```python
from build123d import *

# Parameters (mm, degrees)
F0_R     = 9.4
F1_DEPTH = 3


with BuildPart() as f1:
    # F0 (on Front) → F1 (new body)
    with BuildSketch(Plane.XZ):
        with BuildLine():
            Line((58.8, 11.4), (0, 11.4))
            ThreePointArc((0, 11.4), (-9.870808, 5.703258), (-9.87645, -5.693483))
            Line((-9.87645, -5.693483), (-0.07645, -22.693483))
            Line((-0.07645, -22.693483), (19.523115, -56.692727))
            Line((19.523115, -56.692727), (29.322897, -73.692349))
            ThreePointArc((29.322897, -73.692349), (33.496089, -77.869674), (39.199347, -79.398866))
            Line((39.199347, -79.398866), (156.799347, -79.398866))
            ThreePointArc((156.799347, -79.398866), (166.670155, -73.702124), (166.675796, -62.305384))
            Line((166.675796, -62.305384), (127.47645, 5.693483))
            ThreePointArc((127.47645, 5.693483), (123.303258, 9.870808), (117.6, 11.4))
            Line((117.6, 11.4), (98, 11.4))
            Line((98, 11.4), (58.8, 11.4))
        make_face()
        with Locations((39.199347, -67.998866)):
            Circle(F0_R, mode=Mode.SUBTRACT)
        with Locations((58.799347, -67.998866)):
            Circle(F0_R, mode=Mode.SUBTRACT)
        with Locations((78.399347, -67.998866)):
            Circle(F0_R, mode=Mode.SUBTRACT)
        with Locations((29.399564, -50.999244)):
            Circle(F0_R, mode=Mode.SUBTRACT)
        with Locations((19.599782, -33.999622)):
            Circle(F0_R, mode=Mode.SUBTRACT)
        with Locations((48.999564, -50.999244)):
            Circle(F0_R, mode=Mode.SUBTRACT)
        with Locations((68.599564, -50.999244)):
            Circle(F0_R, mode=Mode.SUBTRACT)
        with Locations((39.199782, -33.999622)):
            Circle(F0_R, mode=Mode.SUBTRACT)
        with Locations((58.799782, -33.999622)):
            Circle(F0_R, mode=Mode.SUBTRACT)
        with Locations((97.999347, -67.998866)):
            Circle(F0_R, mode=Mode.SUBTRACT)
        with Locations((117.599347, -67.998866)):
            Circle(F0_R, mode=Mode.SUBTRACT)
        with Locations((137.199347, -67.998866)):
            Circle(F0_R, mode=Mode.SUBTRACT)
        with Locations((156.799347, -67.998866)):
            Circle(F0_R, mode=Mode.SUBTRACT)
        with Locations((88.199564, -50.999244)):
            Circle(F0_R, mode=Mode.SUBTRACT)
        with Locations((107.799564, -50.999244)):
            Circle(F0_R, mode=Mode.SUBTRACT)
        with Locations((78.399782, -33.999622)):
            Circle(F0_R, mode=Mode.SUBTRACT)
        with Locations((97.999782, -33.999622)):
            Circle(F0_R, mode=Mode.SUBTRACT)
        with Locations((117.599782, -33.999622)):
            Circle(F0_R, mode=Mode.SUBTRACT)
        with Locations((127.399564, -50.999244)):
            Circle(F0_R, mode=Mode.SUBTRACT)
        with Locations((146.999564, -50.999244)):
            Circle(F0_R, mode=Mode.SUBTRACT)
        with Locations((137.199782, -33.999622)):
            Circle(F0_R, mode=Mode.SUBTRACT)
        with BuildLine():
            ThreePointArc((9.8, -26.4), (5.097314, -25.139087), (1.656261, -21.694626))
            ThreePointArc((1.656261, -21.694626), (7.370097, -7.919495), (19.2, -17))
            ThreePointArc((19.2, -17), (16.446804, -23.646804), (9.8, -26.4))
        make_face(mode=Mode.SUBTRACT)
        with Locations((29.4, -17)):
            Circle(F0_R, mode=Mode.SUBTRACT)
        with Locations((49, -17)):
            Circle(F0_R, mode=Mode.SUBTRACT)
        with BuildLine():
            ThreePointArc((76.743739, -12.305374), (77.680505, -14.570097), (78, -17))
            ThreePointArc((78, -17), (75.246804, -23.646804), (68.6, -26.4))
            ThreePointArc((68.6, -26.4), (60.460913, -12.297314), (76.743739, -12.305374))
        make_face(mode=Mode.SUBTRACT)
        with BuildLine():
            ThreePointArc((0, 9.4), (6.646804, 6.646804), (9.4, 0))
            ThreePointArc((9.4, 0), (2.429903, -9.080505), (-8.143739, -4.694626))
            ThreePointArc((-8.143739, -4.694626), (-8.139087, 4.702686), (0, 9.4))
        make_face(mode=Mode.SUBTRACT)
        with BuildLine():
            ThreePointArc((29, 0), (12.953196, -6.646804), (19.6, 9.4))
            ThreePointArc((19.6, 9.4), (26.246804, 6.646804), (29, 0))
        make_face(mode=Mode.SUBTRACT)
        with BuildLine():
            ThreePointArc((48.6, 0), (32.553196, -6.646804), (39.2, 9.4))
            ThreePointArc((39.2, 9.4), (45.846804, 6.646804), (48.6, 0))
        make_face(mode=Mode.SUBTRACT)
        with BuildLine():
            ThreePointArc((68.2, 0), (52.153196, -6.646804), (58.8, 9.4))
            ThreePointArc((58.8, 9.4), (63.502686, 8.139087), (66.943739, 4.694626))
            ThreePointArc((66.943739, 4.694626), (67.880505, 2.429903), (68.2, 0))
        make_face(mode=Mode.SUBTRACT)
        with Locations((88.2, -17)):
            Circle(F0_R, mode=Mode.SUBTRACT)
        with Locations((107.8, -17)):
            Circle(F0_R, mode=Mode.SUBTRACT)
        with Locations((127.4, -17)):
            Circle(F0_R, mode=Mode.SUBTRACT)
        with Locations((78.4, 0)):
            Circle(F0_R, mode=Mode.SUBTRACT)
        with Locations((98, 0)):
            Circle(F0_R, mode=Mode.SUBTRACT)
        with Locations((117.6, 0)):
            Circle(F0_R, mode=Mode.SUBTRACT)
    extrude(amount=F1_DEPTH)


solid = f1.part
```
CAD build for the part. Positions are in the model's coordinates, mm. Coordinates: 2 decimals unless noted, no trailing zeros. Order: outer loops, then holes, each group sorted by start corner. A loop starts at its lowest first (then second) coordinate and runs counter-clockwise, first axis right, second up. Notation, with made-up numbers: (48, 83.25) - (82, 83.25) arc R17 ccw to (82, 96.25) - close; hole circle Ø7 at (18, 9.25). An arc over 180 degrees is marked (long way). Answer in a Markdown table with one row per item.
1. Pull direction Z, two halves, no side cores. Call faces 1 (the face through (28.18, -1.48, -41.68)), 2 (the face through (-9.786, -1.479, 5.847)), 3 (the face through (123.376, -1.479, 9.829)): +Z half, -Z half, draft (parallel to the pull), parting line (faces both ways), or undercut.
Answer:
| item | result |
|---|---|
| face 1 | undercut |
| face 2 | parting line |
| face 3 | +Z half |
2. Drill centre lines: L1, parallel to Z at x = 98, y = -0.85; L2, parallel to Z at x = 121, y = -2.5; L3, parallel to Z at x = 145, y = -0.4. Where is each one in solid material? Low to high. Write a range as from..to.
Answer:
| item | result |
|---|---|
| L1 | -79.4..-77.4, -58.6..-43.4, -24.6..-9.4, 9.4..11.4 |
| L2 | -79.4..-76.76, -59.24..-57.88, -44.11..-42.76, -25.24..-23.88, -10.12..-8.76, 8.76..10.88 |
| L3 | -79.4..-73.24, -62.75..-60.18, -41.81..-39.25, -28.75..-24.7 |
3. Slice it at B-B, the plane x = 131. List the corners of the cut face in (y, z).
Answer:
| item | result |
|---|---|
| outline | (-3, -79.4) - (0, -79.4) - (0, -75.06) - (-3, -75.06) - close; (-3, -60.93) - (0, -60.93) - (0, -59.68) - (-3, -59.68) - close; (-3, -42.32) - (0, -42.32) - (0, -41.07) - (-3, -41.07) - close; (-3, -26.93) - (0, -26.93) - (0, -25.68) - (-3, -25.68) - close; (-3, -8.32) - (0, -8.32) - (0, -0.42) - (-3, -0.42) - close |
4. Slice it at C-C, the plane z = -3. Give the number of separate pieces and of enclosed holes in the cut face, then the cut area to 3 significant figures.
Answer:
| item | result |
|---|---|
| separate pieces | 8 |
| enclosed holes | 0 |
| area | 56.3 mm² |
5. Slice it at D-D, the plane x = 152. List the corners of the cut face in (y, z), then the cut area to 3 significant figures.
Answer:
| item | result |
|---|---|
| outline | (-3, -79.4) - (0, -79.4) - (0, -76.08) - (-3, -76.08) - close; (-3, -59.92) - (0, -59.92) - (0, -58.96) - (-3, -58.96) - close; (-3, -43.04) - (0, -43.04) - (0, -36.85) - (-3, -36.85) - close |
| area | 31.4 mm² |
6. Slice it at A-A, the plane x = 64. List the corners of the cut face in (y, z).
Answer:
| item | result |
|---|---|
| outline | (-3, -79.4) - (0, -79.4) - (0, -75.83) - (-3, -75.83) - close; (-3, -60.17) - (0, -60.17) - (0, -59.2) - (-3, -59.2) - close; (-3, -42.8) - (0, -42.8) - (0, -41.83) - (-3, -41.83) - close; (-3, -26.17) - (0, -26.17) - (0, -25.2) - (-3, -25.2) - close; (-3, -8.8) - (0, -8.8) - (0, -7.83) - (-3, -7.83) - close; (-3, 7.83) - (0, 7.83) - (0, 11.4) - (-3, 11.4) - close |
7. Flat gauge pins, fed straight in: P1, Ø11.5, axis at x = 78.4, z = -34, coming from the -Y side; P2, Ø1.5, axis at x = 26.5, y = -1.5, coming from the -Z side; P3, Ø1, axis at y = -2, z = -23.5, coming from the +X side. Where does each tip first touch, or does it go through?
Answer:
| item | result |
|---|---|
| P1 | through |
| P2 | z = -70.1 |
| P3 | x = 144.59 |
